The model under review builds one solid part; all positions refer to its coordinate system, in mm. A direction names the side the tool comes from. Coordinates: 2 decimals unless noted, no trailing zeros. Loops run counter-clockwise (first coordinate to the right, second up) from the corner with the lowest first, then second, coordinate; pieces in that order, holes last. Notation, with made-up numbers: M -20.5,62.25 L -12.5,62.25 A6 cw -12.5,70.25 Z; hole C 0,41.5 d1. An arc over 180 degrees is marked long. One line per item, written item: value.
```python
from build123d import *

# Parameters (mm, degrees)
BOSS_EXTRUDE1_DEPTH = 654.07286
CUT_EXTRUDE1_REACH  = 5.175
SKETCH2_R           = 2.54
SKETCH3_W           = 34.925
SKETCH3_H           = 49.342597017
CUT_EXTRUDE2_DEPTH  = 4.175


with BuildPart() as part:
    # Sketch1 → Boss-Extrude1 (new body)
    with BuildSketch(Plane(origin=(0, 0, 0), x_dir=(0, 0, -1), z_dir=(1, 0, 0))):
        with BuildLine():
            Line((3.175, 3.175), (16.51, 3.175))
            ThreePointArc((16.51, 3.175), (18.306051224, 2.431051224), (19.05, 0.635))
            Line((19.05, 0.635), (19.05, 0))
            Line((19.05, 0), (0, 0))
            Line((0, 0), (0, 19.05))
            Line((0, 19.05), (0.635, 19.05))
            ThreePointArc((0.635, 19.05), (2.431051224, 18.306051224), (3.175, 16.51))
            Line((3.175, 16.51), (3.175, 3.175))
        make_face()
    extrude(amount=BOSS_EXTRUDE1_DEPTH)

    # Sketch2 → Cut-Extrude1 (cut, up to next)
    with BuildSketch(Plane(origin=(0, 3.175, 0), x_dir=(1, 0, 0), z_dir=(0, 1, 0)), mode=Mode.PRIVATE) as cut_extrude1_sk1:
        with Locations((641.37286, 9.8425)):
            Circle(SKETCH2_R)
    cut_extrude1_tool1 = extrude(cut_extrude1_sk1.sketch, amount=-CUT_EXTRUDE1_REACH, mode=Mode.PRIVATE) & part.part
    add(cut_extrude1_tool1.solids().sort_by_distance((641.37286, 3.175, -9.8425))[0], mode=Mode.SUBTRACT)
    # Sketch2 → Cut-Extrude1 (cut, up to next)
    with BuildSketch(Plane(origin=(0, 3.175, 0), x_dir=(1, 0, 0), z_dir=(0, 1, 0)), mode=Mode.PRIVATE) as cut_extrude1_sk2:
        with Locations((12.7, 9.8425)):
            Circle(SKETCH2_R)
    cut_extrude1_tool2 = extrude(cut_extrude1_sk2.sketch, amount=-CUT_EXTRUDE1_REACH, mode=Mode.PRIVATE) & part.part
    add(cut_extrude1_tool2.solids().sort_by_distance((12.7, 3.175, -9.8425))[0], mode=Mode.SUBTRACT)

    # Sketch3 → Cut-Extrude2 (cut, through all)
    with BuildSketch(Plane(origin=(0, 0, -3.175), x_dir=(-1, 0, 0), z_dir=(0, 0, -1))):
        with Locations((-334.98536, 27.846298508)):
            Rectangle(SKETCH3_W, SKETCH3_H)
    extrude(amount=-CUT_EXTRUDE2_DEPTH, mode=Mode.SUBTRACT)


solid = part.part
```
(1) Add section A-A on y = 6.5. State the section outline as (x, z) points (3 decimals), then the cut area to 3 significant figures.
Checks:
outline: M 0,-3.175 L 317.523,-3.175 L 317.523,0 L 0,0 Z; M 352.448,-3.175 L 654.073,-3.175 L 654.073,0 L 352.448,0 Z
area: 1,970 mm^2
(2) To check wall thickness, follow L1, parallel to Z at x = 12.7, y = 1.05; L2, parallel to Y at x = 381, z = -14.25 (3 decimals); L3, parallel to X at y = 1.5, z = -11.5. State the ranges of each line that lie inside material, in increasing order. Write a range as [from, to].
Checks:
L1: [-19.02, -12.38], [-7.3, 0]
L2: [0, 3.175]
L3: [0, 10.78], [14.62, 639.45], [643.3, 654.07]
(3) Add section B-B on x = 558.5. State the section outline as (y, z) points (3 decimals), then the cut area to 3 significant figures.
Checks:
outline: M 0,-19.05 L 0.635,-19.05 A2.54 ccw 3.175,-16.51 L 3.175,-3.175 L 16.51,-3.175 A2.54 ccw 19.05,-0.635 L 19.05,0 L 0,0 Z
area: 108 mm^2
(4) Insertion check: pin 1 Ø4.5 at (x, z) = (12.7, -9.84) entering from +Y; pin 2 Ø8.5 at (x, z) = (295.5, -7) entering from +Y; pin 3 Ø5 at (x, z) = (65.5, -4.5) entering from +Y; pin 4 Ø10.5 at (x, y) = (170.5, 8.5) entering from -Z (3 decimals). Each pin has a flat end and moves straight along its axis. Give the tip position at first contact, or say it passes through.
Checks:
pin 1: through
pin 2: y = 17.92
pin 3: y = 18.65
pin 4: z = -3.175
(5) Tool access review of faces 1 (the face through (654.073, 6, -3)), 2 (the face through (501, 10, -3.175)): name each direction out of +Z, -Z, +X, -X, +Y, -Y from which nothing blocks a thin tool from reaching the whole face with its end or side.
Checks:
face 1: +Z, -Z, +X, +Y, -Y
face 2: -Z, +X, -X, +Y
